Read the model definition and answer for the solid it produces. Units are mm, in the model's axes. A direction names the side the tool comes from. Round coordinates to 2 decimals unless told otherwise and drop trailing zeros. Order: outer loops, then holes, each group sorted by start corner. A loop starts at its lowest first (then second) coordinate and runs counter-clockwise, first axis right, second up. Notation, with made-up numbers: (45, -7) -> (60, -7) arc R29 cw to (60, 31) -> close; hole circle Ø2 at (28.25, 79). An arc over 180 degrees is marked (long way). Answer as a JSON object with one key per item and string values. Group by question number.
Item 1: Section B-B, the plane x = 0 is taken. Write down the section's boundary in (y, z).
Item 2: Consider probe 1 along Z at (x, y) = (-2, 1.5); probe 2 along Y at (x, z) = (-5.5, 16.5); probe 3 along X at (y, z) = (2.25, 1.5). Determine where each line is inside the solid, lowest interval first. Write a range as from..to.
Item 3: Section A-A, the plane z = 1.5 is taken. Write down the section's boundary in (x, y), plus the area to 3 significant figures.
Item 4: Section D-D, the plane x = 4.5 is taken. Write down the section's boundary in (y, z), plus the area to 3 significant figures.
Item 5: Given P1, Ø1.5, axis at x = -11, z = 7.5, coming from the +Y side; P2, Ø12, axis at x = 5.5, z = 10, coming from the -Y side; P3, Ø5, axis at y = 6.5, z = 4, coming from the -X side; P4, Ø1.2, axis at x = 14.5, y = -1, coming from the -Z side, each flat-ended and moving along its own axis, determine where each tip first touches the part or whether it passes through.
Item 6: Section C-C, the plane z = 16.5 is taken. Write down the section's boundary in (x, y), plus the area to 3 significant figures.
Item 7: For faces 4 (the flat face through (0, 5, 16)), 5 (the flat face through (0, 0, 10)), 6 (the flat face through (-15, 0, 15)), determine the directions among +Z, -Z, +X, -X, +Y, -Y from which every point of the face is accessible in a straight line to the end or side of a thin tool.
Item 8: The mould has two halves that part along Y. Classify faces 1 (the flat face through (3.9, 0, 5)), 2 (the flat face through (0, 0, 20)), 3 (the flat face through (0, -5, 16)): pulls with the +Y half, pulls with the -Y half, needs draft (parallel to the pull), parting line crosses it, or undercut.
from build123d import *

# Parameters (mm, degrees)
F0_R         = 8.5154328933
F0_W         = 7.8
F0_H         = 7.8
F1_DEPTH     = 10
F2_W         = 7.8
F2_H         = 7.8
F3_DEPTH     = 10
F4_T4_DEPTH  = 38.7858764479
F4_S5_R      = 8.5154328933
F4_T6_DEPTH  = 21
F4_T10_DEPTH = 38.7858764479
F4_S11_R     = 8.5154328933
F4_T12_DEPTH = 21
F4_T16_ANGLE = 120.0675682876
F4_T21_ANGLE = 240.167490735
F4_T27_ANGLE = 120.0675682876


# Not quite as in the source:
# - a fillet or chamfer that OpenCascade refuses, or shapes differently, is made with other operations: its cross-section is extruded or revolved along the edge and cut away or added
# - two fillets or chamfers of one size are made in one step


with BuildPart() as f1:
    # F0 (on Top) → F1 (new body)
    with BuildSketch(Plane.XY):
        Circle(F0_R)
        Rectangle(F0_W, F0_H, mode=Mode.SUBTRACT)
    extrude(amount=F1_DEPTH)

    # F2 (on face) → F3 (join)
    with BuildSketch(Plane.XY.offset(10)):
        with BuildLine():
            Line((6.892938224, 5), (-6.892938224, 5))
            ThreePointArc((-6.892938224, 5), (-8.5154328933, 0), (-6.892938224, -5))
            Line((-6.892938224, -5), (6.892938224, -5))
            ThreePointArc((6.892938224, -5), (8.0996589509, -2.6283306942), (8.5154328933, 0))
            ThreePointArc((8.5154328933, 0), (8.0996589509, 2.6283306942), (6.892938224, 5))
        make_face()
        Rectangle(F2_W, F2_H, mode=Mode.SUBTRACT)
        with BuildLine():
            Line((-6.892938224, 5), (-15, 5))
            Line((-15, 5), (-15, -5))
            Line((-15, -5), (-6.892938224, -5))
            ThreePointArc((-6.892938224, -5), (-8.5154328933, 0), (-6.892938224, 5))
        make_face()
        with BuildLine():
            Line((15, 5), (6.892938224, 5))
            ThreePointArc((6.892938224, 5), (8.0996589509, 2.6283306942), (8.5154328933, 0))
            ThreePointArc((8.5154328933, 0), (8.0996589509, -2.6283306942), (6.892938224, -5))
            Line((6.892938224, -5), (15, -5))
            Line((15, -5), (15, 5))
        make_face()
        Rectangle(F2_W, F2_H)
    extrude(amount=F3_DEPTH)

    # F4: fillet of radius 5 on 5 edges, made by hand


with BuildPart() as f4_tool2:
    # F4_s3 → F4_t4 (new body)
    with BuildSketch(Plane.YZ.offset(-19.392938224)):
        with BuildLine():
            ThreePointArc((-10, 10), (-6.4644660941, 11.4644660941), (-5, 15))
            Line((-5, 15), (-5, 10))
            Line((-5, 10), (-10, 10))
        make_face()
    extrude(amount=F4_T4_DEPTH)

    # F4_s5 → F4_t6 (intersect, symmetric)
    with BuildSketch(Plane.XY.offset(12.5)):
        Circle(F4_S5_R)
    extrude(amount=F4_T6_DEPTH, both=True, mode=Mode.INTERSECT)


with BuildPart() as f1_1:
    add(f1.part)

    # F4_t1: union F4_tool2
    add(f4_tool2.part)


with BuildPart() as f4_tool8:
    # F4_s9 → F4_t10 (new body)
    with BuildSketch(Plane.YZ.offset(19.392938224)):
        with BuildLine():
            ThreePointArc((10, 10), (6.4644660941, 11.4644660941), (5, 15))
            Line((5, 15), (5, 10))
            Line((5, 10), (10, 10))
        make_face()
    extrude(amount=-F4_T10_DEPTH)

    # F4_s11 → F4_t12 (intersect, symmetric)
    with BuildSketch(Plane.XY.offset(12.5)):
        Circle(F4_S11_R)
    extrude(amount=F4_T12_DEPTH, both=True, mode=Mode.INTERSECT)


with BuildPart() as f1_2:
    add(f1_1.part)

    # F4_t7: union F4_tool8
    add(f4_tool8.part)


with BuildPart() as f4_tool14:
    # F4_s15 → F4_t16 (revolve)
    with BuildSketch(Plane(origin=(0, 0, 0), x_dir=(0, 0, 1), z_dir=(-0.8654351572, 0.5010209464, 0))):
        with BuildLine():
            ThreePointArc((5, -8.5154328933), (8.5355339059, -9.9798989873), (10, -13.5154328933))
            Line((10, -13.5154328933), (10, -8.5154328933))
            Line((10, -8.5154328933), (5, -8.5154328933))
        make_face()
    revolve(axis=Axis((0, 0, 10), (0, 0, 1)), revolution_arc=F4_T16_ANGLE)

    split(bisect_by=Plane.XZ.offset(5), keep=Keep.BOTTOM)


with BuildPart() as f1_3:
    add(f1_2.part)

    # F4_t13: union F4_tool14
    add(f4_tool14.part)


with BuildPart() as f4_tool19:
    # F4_s20 → F4_t21 (revolve)
    with BuildSketch(Plane(origin=(0, 0, 0), x_dir=(0, 0, 1), z_dir=(0.8652936628, -0.5012652762, 0))):
        with BuildLine():
            ThreePointArc((5, -8.5154328933), (8.5355339059, -9.9798989873), (10, -13.5154328933))
            Line((10, -13.5154328933), (10, -8.5154328933))
            Line((10, -8.5154328933), (5, -8.5154328933))
        make_face()
    revolve(axis=Axis((0, 0, 10), (0, 0, 1)), revolution_arc=F4_T21_ANGLE)

    split(bisect_by=Plane.XZ.offset(-5), keep=Keep.TOP)

    split(bisect_by=Plane.XZ.offset(5), keep=Keep.BOTTOM)


with BuildPart() as f1_4:
    add(f1_3.part)

    # F4_t18: union F4_tool19
    add(f4_tool19.part)


with BuildPart() as f4_tool25:
    # F4_s26 → F4_t27 (revolve)
    with BuildSketch(Plane.XZ):
        with BuildLine():
            ThreePointArc((8.5154328933, 5), (9.9798989873, 8.5355339059), (13.5154328933, 10))
            Line((13.5154328933, 10), (8.5154328933, 10))
            Line((8.5154328933, 10), (8.5154328933, 5))
        make_face()
    revolve(axis=Axis((0, 0, 10), (0, 0, 1)), revolution_arc=F4_T27_ANGLE)

    split(bisect_by=Plane.XZ.offset(-5), keep=Keep.TOP)


with BuildPart() as f1_5:
    add(f1_4.part)

    # F4_t24: union F4_tool25
    add(f4_tool25.part)


solid = f1_5.part
Values found:
{
 "1": {"outline": "(-8.52, 0) -> (-3.9, 0) -> (-3.9, 10) -> (3.9, 10) -> (3.9, 0) -> (8.52, 0) -> (8.52, 10.23) arc R5 cw to (5, 15) -> (5, 20) -> (-5, 20) -> (-5, 15) arc R5 cw to (-8.52, 10.23) -> close"},
 "2": {"probe 1": "10..20", "probe 2": "-5..5", "probe 3": "-8.21..-3.9, 3.9..8.21"},
 "3": {"outline": "circle Ø17.03 at (0, 0); hole (-3.9, -3.9) -> (3.9, -3.9) -> (3.9, 3.9) -> (-3.9, 3.9) -> close", "area": "167 mm2"},
 "4": {"outline": "(-7.23, 0) -> (7.23, 0) -> (7.23, 10.84) arc R5 cw to (5, 15) -> (5, 20) -> (-5, 20) -> (-5, 15) arc R5 cw to (-7.23, 10.84) -> close", "area": "254 mm2"},
 "5": {"P1": "through", "P2": "y = -8.52", "P3": "x = -7.52", "P4": "z = 10"},
 "6": {"outline": "(-15, -5) -> (15, -5) -> (15, 5) -> (-15, 5) -> close", "area": "300 mm2"},
 "7": {"face 4": "+Z, +Y", "face 5": "-Z", "face 6": "+Z, -Z, -X, +Y, -Y"},
 "8": {"face 1": "undercut", "face 2": "needs draft", "face 3": "pulls with the -Y half"}
}
